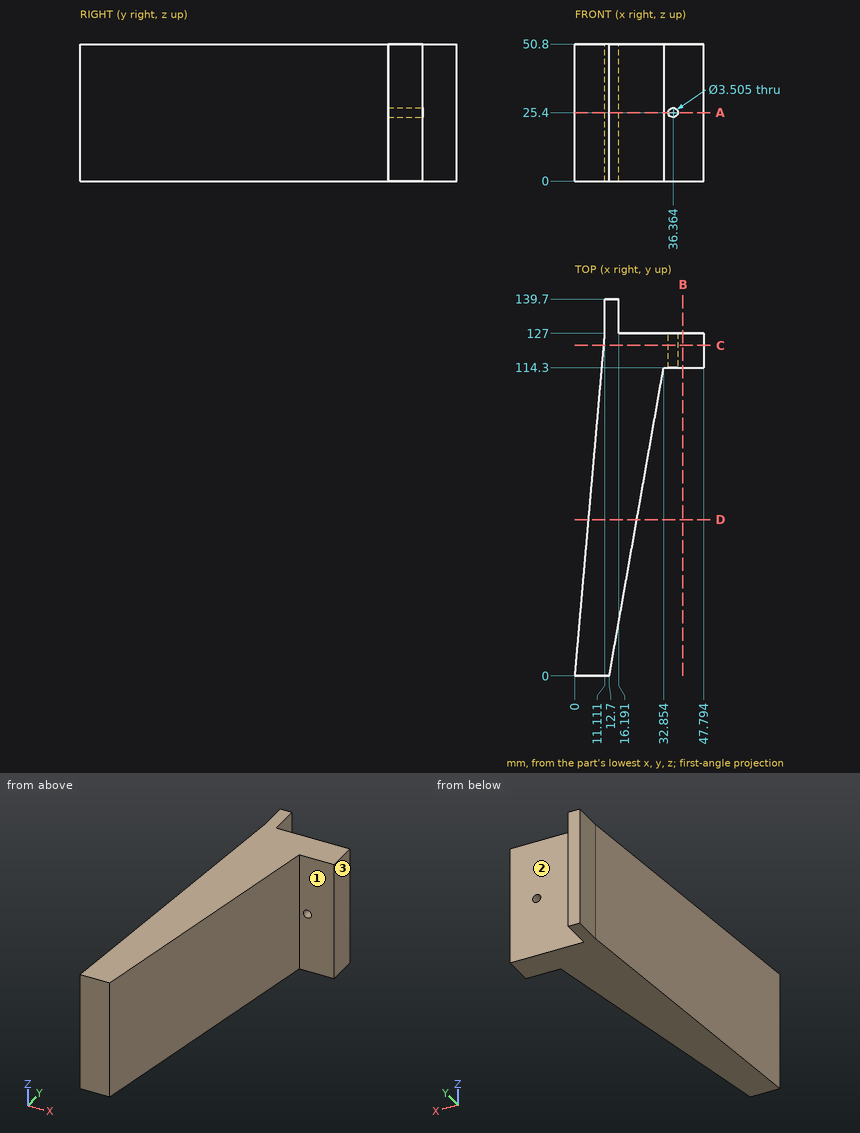
Job drawing, mm, ordinate dimensions from the low corner. One solid piece. A direction names the side the tool comes from. Coordinates: 2 decimals unless noted, no trailing zeros. Loops run counter-clockwise (first coordinate to the right, second up) from the corner with the lowest first, then second, coordinate; pieces in that order, holes last. Notation, with made-up numbers: (24, -34) - (43, -34) arc R27 ccw to (43, 1) - close; hole circle Ø1 at (55.25, 14.25). An arc over 180 degrees is marked (long way). Answer as a JSON object with one key per item and string values. Group by question number.
(1) Probe line 1 along Y through (x, z) = (39, 48.5); line 2 along X through (y, z) = (118, 25.4); line 3 along X through (y, z) = (109, 5.5) (1 decimal). List the from-to ranges inside material, lowest first.
(2) Cut at B-B (x = 40). Give the cut face in (y, z).
(3) Cut at C-C (y = 122.5). Give the cut face in (x, z) (1 decimal).
(4) Tool access for the marked faces 1, 2 and 3: list every direction of +Z, -Z, +X, -X, +Y, -Y with a clear straight run to the whole face (end or side of a thin tool).
(5) Cut at A-A (z = 25.4). Give the cut face in (x, y) (1 decimal).
(6) Cut at D-D (y = 58). Give the cut face in (x, z) (1 decimal).
(7) Flat gauge pins, fed straight in: pin 1 (4 mm diameter, centred on y = 133.5, z = 22.5, fed in from -X); pin 2 (8 mm diameter, centred on x = 24.5, z = 34.5, fed in from +Y); pin 3 (4 mm diameter, centred on y = 116.5, z = 26, fed in from -X). Where does each tip first touch, or does it go through?
Geometry says:
{
 "1": {"line 1": "y = 114.3 to 127", "line 2": "x = 10.32 to 34.61, 38.12 to 47.79", "line 3": "x = 9.5 to 31.9"},
 "2": {"outline": "(114.3, 0) - (127, 0) - (127, 50.8) - (114.3, 50.8) - close"},
 "3": {"outline": "(10.7, 0) - (47.8, 0) - (47.8, 50.8) - (10.7, 50.8) - close; hole circle Ø3.5 at (36.4, 25.4)"},
 "4": {"face 1": "+Z, -Z, +X, -Y", "face 2": "+Z, -Z, +X, +Y", "face 3": "+Z, -Z, +X, +Y, -Y"},
 "5": {"outline": "(0, 0) - (12.7, 0) - (32.9, 114.3) - (34.6, 114.3) - (34.6, 127) - (16.2, 127) - (16.2, 139.7) - (11.1, 139.7) - (11.1, 127) - close; (38.1, 114.3) - (47.8, 114.3) - (47.8, 127) - (38.1, 127) - close"},
 "6": {"outline": "(5.1, 0) - (22.9, 0) - (22.9, 50.8) - (5.1, 50.8) - close"},
 "7": {"pin 1": "stops at x = 11.11", "pin 2": "stops at y = 127", "pin 3": "stops at x = 10.02"}
}
